Geometry check sheet. Reference: the model listing, model coordinates, mm. Face numbers are marked on the shaded views. A direction names the side the tool comes from. Round coordinates to 2 decimals unless told otherwise and drop trailing zeros. Loops run counter-clockwise (first coordinate to the right, second up) from the corner with the lowest first, then second, coordinate; pieces in that order, holes last.
Autodesk Inventor part; units mm, degrees
ref_plane "YZ Plane" through (0, 0, 0) normal (1, 0, 0) x (0, 1, 0)
ref_plane "XZ Plane" through (0, 0, 0) normal (0, 1, 0) x (-1, 0, 0)
ref_plane "XY Plane" through (0, 0, 0) normal (0, 0, 1) x (1, 0, 0)
sketch "Sketch1" plane through (0, 0, 0) normal (0, 1, 0) x (-1, 0, 0)
  circle A0 centre (0, 0) radius 6.3
  dimension "d0" = 12.6
extrude "Extrusion1" add sketch "Sketch1" along normal mid plane 113.75
sketch "Sketch2" plane through (0, 0, 0) normal (1, 0, 0) x (0, 1, 0)
  line L0 (56.875, -6.3) -> (56.875, 6.3)
  line L1 (-56.875, -6.3) -> (56.875, -6.3)
  line L2 (56.875, 6.3) -> (45.245, 6.3)
  line L3 (45.245, 6.3) -> (45.245, -6.3)
  line L4 (45.245, -6.3) -> (56.875, -6.3)
  line L5 (56.875, -6.3) -> (56.875, 6.3)
  line L6 (56.875, 0) -> (51.875, 0)
  circle A0 centre (51.875, 0) radius 3
  point P0 (0, 0)
  dimension "d3" = 11.63
  dimension "d7" = 5
  dimension "d8" = 6
sketch "Sketch3" plane through (0, 56.875, 0) normal (0, 1, 0) x (1, 0, 0)
  circle A0 centre (0, 0) radius 6.3
  line L0 (2, -5.9741) -> (-2, -5.9741)
  line L1 (-2, -5.9741) -> (-2, 5.9741)
  line L2 (-2, 5.9741) -> (2, 5.9741)
  line L3 (2, 5.9741) -> (2, -5.9741)
  line L4 (2, -5.9741) -> (-2, 5.9741) construction
  line L5 (-2, -5.9741) -> (2, 5.9741) construction
  dimension "d4" = 4
extrude "Extrusion2" cut sketch "Sketch3" against normal blind 11.63 contours A0 L3 | L1 A0
extrude "Extrusion3" cut sketch "Sketch2" against normal mid plane 11.63 contours A0
sketch "Sketch4" plane through (0, -56.875, 0) normal (0, -1, 0) x (1, 0, 0)
  circle A0 centre (0, 0) radius 7.25
  dimension "d11" = 14.5
extrude "Extrusion4" add sketch "Sketch4" against normal blind 10
properties part number "vastago"
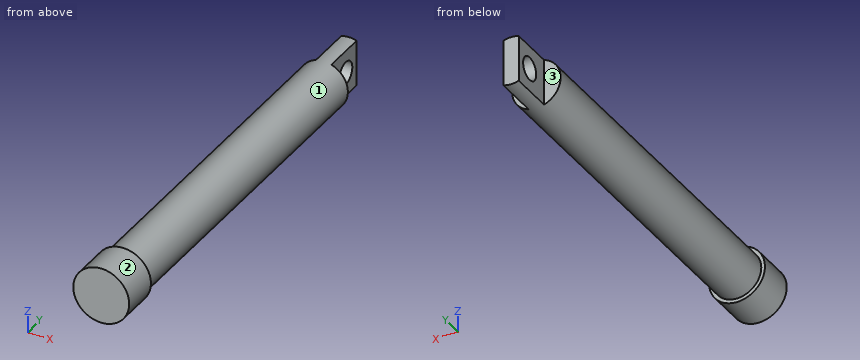
1) Scan lines: line 1 along Y through (x, z) = (-2.25, 1.5) (3 decimals); line 2 along Z through (x, y) = (-2, 0); line 3 along Y through (x, z) = (-0.75, 2) (3 decimals). Record each from-to range of solid material in increasing order.
Report:
line 1: y = -56.875 to 45.245
line 2: z = -5.97 to 5.97
line 3: y = -56.875 to 49.639, 54.111 to 56.875
2) Sectioned sample at C-C, the plane y = -13.5. Record the cut outline in (x, z).
Report:
outline: circle Ø12.6 at (0, 0)
3) Gauge pin test, flat ends, axial feed: pin 1 (4 mm diameter, centred on y = 26.5, z = -4.5, fed in from -X); pin 2 (3.5 mm diameter, centred on y = 52.5, z = 2.5, fed in from -X); pin 3 (1.3 mm diameter, centred on x = -4, z = 2, fed in from +Y) (3 decimals). Record the tip position at first contact, or that the pin passes through.
Report:
pin 1: stops at x = -5.78
pin 2: stops at x = -2
pin 3: stops at y = 45.245
4) Sectioned sample at D-D, the plane z = 4.5. Record the cut outline in (x, y) (3 decimals).
Report:
outline: (-5.684, -56.875) - (5.684, -56.875) - (5.684, -46.875) - (4.409, -46.875) - (4.409, 45.245) - (2, 45.245) - (2, 56.875) - (-2, 56.875) - (-2, 45.245) - (-4.409, 45.245) - (-4.409, -46.875) - (-5.684, -46.875) - close
5) Sectioned sample at A-A, the plane z = 0. Record the cut outline in (x, y) (3 decimals), then the cut area to 3 significant figures.
Report:
outline: (-7.25, -56.875) - (7.25, -56.875) - (7.25, -46.875) - (6.3, -46.875) - (6.3, 45.245) - (2, 45.245) - (2, 48.875) - (-2, 48.875) - (-2, 45.245) - (-6.3, 45.245) - (-6.3, -46.875) - (-7.25, -46.875) - close; (-2, 54.875) - (2, 54.875) - (2, 56.875) - (-2, 56.875) - close
area: 1,330 mm2
6) Access from +Z, -Z, +X, -X, +Y, -Y to the whole of each face (thin tool, end or side, straight path). Record for the marked faces 1, 2 and 3.
Report:
face 1: +Y
face 2: +Y, -Y
face 3: +Z, -Z, -X, +Y
7) Sectioned sample at B-B, the plane x = 0. Record the cut outline in (y, z) (3 decimals), then the cut area to 3 significant figures.
Report:
outline: (-56.875, -7.25) - (-46.875, -7.25) - (-46.875, -6.3) - (56.875, -6.3) - (56.875, 6.3) - (-46.875, 6.3) - (-46.875, 7.25) - (-56.875, 7.25) - close; hole circle Ø6 at (51.875, 0)
area: 1,420 mm2
